Verification items for the finished model (mm, model axes). A direction names the side the tool comes from. Round coordinates to 2 decimals unless told otherwise and drop trailing zeros. Order: outer loops, then holes, each group sorted by start corner. A loop starts at its lowest first (then second) coordinate and runs counter-clockwise, first axis right, second up. Notation, with made-up numbers: (62, 58) -> (73, 58) arc R10 cw to (73, 72) -> close; hole circle Ø7 at (-38.5, -31.75). An arc over 180 degrees is marked (long way). Put each result on its own line as item: value.
```python
from build123d import *

# Parameters (mm, degrees)
SKETCH2_R           = 6.858
EXTRUDE1_DEPTH      = 13.273264
EXTRUDE1_DRAFT      = -1.783333333
CHAMFER1_SIZE       = 1.002631579
CHAMFER1_SIZE2      = 1.035353254
SKETCH5_R           = 5.1435
EXTRUDE2_DEPTH      = 13.273264
EXTRUDE2_TAPER      = 1.783333333
CHAMFER2_SIZE       = 0.705555556
CHAMFER2_SIZE_2     = 0.728581919
EXTRUDE3_DEPTH      = 3.792361
EXTRUDE3_DEPTH_BACK = 3.792361
SKETCH10_OUTSIDE_W  = 118.396
SKETCH10_OUTSIDE_H  = 121.158
SKETCH10_OUTSIDE_R  = 8.9296875
CUT_EXTRUDE1_DEPTH  = 25.922158813
CUT_EXTRUDE1_DRAFT  = -60
SKETCH11_OUTSIDE_W  = 118.396
SKETCH11_OUTSIDE_H  = 121.158
SKETCH11_OUTSIDE_R  = 8.9296875
CUT_EXTRUDE2_DEPTH  = 25.922158813
CUT_EXTRUDE2_DRAFT  = -60
SKETCH12_R          = 4.6228
CUT_EXTRUDE3_DEPTH  = 13.273265
SKETCH13_R          = 3.4163
CUT_EXTRUDE4_DEPTH  = 37.75596067


with BuildPart() as part:
    # Sketch2 → Extrude1 (with draft: the straight prism first)
    with BuildSketch(Plane(origin=(-3.792361111, 0, 0), x_dir=(0, 0, -1), z_dir=(1, 0, 0))):
        Circle(SKETCH2_R)
    extrude(amount=-EXTRUDE1_DEPTH)
    # Extrude1: the draft: its side faces are tilted about the plane it starts from
    extrude1_sides = [part.faces().sort_by_distance(p)[0] for p in [
        (-10.428993111, 0, 6.858),
    ]]
    draft(extrude1_sides, Plane(origin=(-3.792361111, 0, 0), x_dir=(0, 0, -1), z_dir=(1, 0, 0)), EXTRUDE1_DRAFT)

    # Chamfer1
    chamfer1_edges = [part.edges().sort_by_distance(p)[0] for p in [
        (-17.065625111, 0, 6.444735688),
    ]]
    chamfer1_side = [part.faces().sort_by_distance(p)[0] for p in [
        (-17.065625111, 0, 0),
    ]]
    chamfer(chamfer1_edges, length=CHAMFER1_SIZE, length2=CHAMFER1_SIZE2, reference=chamfer1_side[0])



with BuildPart() as body_2:
    # Sketch5 → Extrude2 (new body)
    with BuildSketch(Plane(origin=(3.792361111, 0, 0), x_dir=(0, 0, -1), z_dir=(1, 0, 0))):
        Circle(SKETCH5_R)
    extrude(amount=EXTRUDE2_DEPTH, taper=EXTRUDE2_TAPER)

    # Chamfer2
    # the kernel refuses this chamfer: 0.728581919, 0.705555556 mm, written as the material it takes off along each edge
    with BuildSketch(Plane(origin=(17.065625111, 0, 0), x_dir=(0, 0, -1), z_dir=(0, 1, 0))) as chamfer2_piece_1:
        Polygon((4.730235688 + CHAMFER2_SIZE * 0.0311200130608, CHAMFER2_SIZE * 0.999515654468), (4.730235688 - CHAMFER2_SIZE_2, 0), (4.730235688, 0), align=None)
    revolve(axis=Axis((17.065625111, 0, 0), (-1, 0, 0)), mode=Mode.SUBTRACT)


with BuildPart() as part_1:
    add(part.part)

    add(body_2.part)  # Revolve1 merges body 2
    # Sketch8 → Revolve1 (revolve)
    with BuildSketch(Plane.XY, mode=Mode.PRIVATE) as revolve1_sk:
        Polygon((0, 6.858), (-3.792361111, 6.858), (-10.476571637, 5.066971187), (-10.476571637, 0), (10.476571637, 0), (10.476571637, 3.352471187), (3.792361111, 5.1435), (0, 5.1435), align=None)
    revolve(revolve1_sk.sketch.rotate(Axis((-17.065625, 0, 0), (1, 0, 0)), 90), axis=Axis((-17.065625, 0, 0), (1, 0, 0)))

    # Sketch9 → Extrude3 (add, two sides: drawn at the far end of the back side and taken through both)
    with BuildSketch(Plane(origin=(0, 0, 0), x_dir=(0, 0, -1), z_dir=(1, 0, 0)).offset(-EXTRUDE3_DEPTH_BACK)):
        Polygon((0, 10.311114964), (-8.9296875, 5.155557482), (-8.9296875, -5.155557482), (0, -10.311114964), (8.9296875, -5.155557482), (8.9296875, 5.155557482), align=None)
    extrude(amount=EXTRUDE3_DEPTH + EXTRUDE3_DEPTH_BACK)


with BuildPart() as cut_extrude1_tool:
    # Sketch10 outside → Cut-Extrude1 (with draft: the straight prism first)
    with BuildSketch(Plane(origin=(3.792361111, 0, 0), x_dir=(0, 0, -1), z_dir=(1, 0, 0))):
        Rectangle(SKETCH10_OUTSIDE_W, SKETCH10_OUTSIDE_H)
        Circle(SKETCH10_OUTSIDE_R, mode=Mode.SUBTRACT)
    extrude(amount=-CUT_EXTRUDE1_DEPTH)
    # Cut-Extrude1: the draft: its side faces are tilted about the plane it starts from
    cut_extrude1_sides = [cut_extrude1_tool.faces().sort_by_distance(p)[0] for p in [
        (-9.168718295, -60.579, 0),
        (-9.168718295, 0, -59.198),
        (-9.168718295, 60.579, 0),
        (-9.168718295, 0, 59.198),
        (-9.168718295, 0, 8.9296875),
    ]]
    draft(cut_extrude1_sides, Plane(origin=(3.792361111, 0, 0), x_dir=(0, 0, -1), z_dir=(1, 0, 0)), CUT_EXTRUDE1_DRAFT)


with BuildPart() as part_2:
    add(part_1.part)

    # Cut-Extrude1: cut by cut_extrude1_tool
    add(cut_extrude1_tool.part, mode=Mode.SUBTRACT)


with BuildPart() as cut_extrude2_tool:
    # Sketch11 outside → Cut-Extrude2 (with draft: the straight prism first)
    with BuildSketch(Plane.ZY.offset(3.792361111)):
        Rectangle(SKETCH11_OUTSIDE_W, SKETCH11_OUTSIDE_H)
        Circle(SKETCH11_OUTSIDE_R, mode=Mode.SUBTRACT)
    extrude(amount=-CUT_EXTRUDE2_DEPTH)
    # Cut-Extrude2: the draft: its side faces are tilted about the plane it starts from
    cut_extrude2_sides = [cut_extrude2_tool.faces().sort_by_distance(p)[0] for p in [
        (9.168718295, -60.579, 0),
        (9.168718295, 0, 59.198),
        (9.168718295, 60.579, 0),
        (9.168718295, 0, -59.198),
        (9.168718295, 0, -8.9296875),
    ]]
    draft(cut_extrude2_sides, Plane.ZY.offset(3.792361111), CUT_EXTRUDE2_DRAFT)


with BuildPart() as part_3:
    add(part_2.part)

    # Cut-Extrude2: cut by cut_extrude2_tool
    add(cut_extrude2_tool.part, mode=Mode.SUBTRACT)

    # Sketch12 → Cut-Extrude3 (cut)
    with BuildSketch(Plane.ZY.offset(17.065625)):
        Circle(SKETCH12_R)
    extrude(amount=-CUT_EXTRUDE3_DEPTH, mode=Mode.SUBTRACT)

    # Sketch13 → Cut-Extrude4 (cut, through all)
    with BuildSketch(Plane(origin=(17.065625, 0, 0), x_dir=(0, 0, -1), z_dir=(1, 0, 0))):
        Circle(SKETCH13_R)
    extrude(amount=-CUT_EXTRUDE4_DEPTH, mode=Mode.SUBTRACT)

    # Cut-Extrude5 cone 1 section (through the dimple's axis) → Cut-Extrude5 (revolve, cut)
    with BuildSketch(Plane(origin=(-3.792361111, 0, 0), x_dir=(0, 0, 1), z_dir=(0, 1, 0))):
        Polygon((0, 0), (4.6228, 0), (0, 5.317923073), align=None)
    revolve(axis=Axis((-3.792361111, 0, 0), (1, 0, 0)), mode=Mode.SUBTRACT)


solid = part_3.part
```
Item 1: Release check for a two-part mould opening along Y. For faces 3 (the face through (-3.6, -9.26, -0.02)), 4 (the face through (-3.6, 4.61, 8.03)), 5 (the face through (-10.52, -2.81, -3.67)) record: pulls with the +Y half, pulls with the -Y half, needs draft (parallel to the pull), parting line crosses it, or undercut.
Geometry check:
face 3: pulls with the -Y half
face 4: pulls with the +Y half
face 5: undercut
Item 2: Depth check by flat-ended pin: pin 1 Ø8 at (y, z) = (5, -5) entering from -X; pin 2 Ø8 at (y, z) = (0, 0) entering from -X; pin 3 Ø1.5 at (x, z) = (5, -1.5) entering from -Y; pin 4 Ø3 at (x, z) = (-5, 6) entering from +Y. Enter the tip coordinate at first touch or a pass-through.
Geometry check:
pin 1: x = -17.07
pin 2: x = -3.08
pin 3: y = -5.05
pin 4: y = 7.35
Item 3: Material ranges on line 1 along Y through (x, z) = (2, 0); line 2 along Z through (x, y) = (4, 0); line 3 along X through (y, z) = (2.75, 7), recorded low to high.
Geometry check:
line 1: -10.31 to -3.42, 3.42 to 10.31
line 2: -5.14 to -3.42, 3.42 to 5.14
line 3: -3.79 to 3.79
Item 4: Tool access check on faces 1 (the face through (3.792, -4, -4)), 2 (the face through (0, 8, 4)). Record the directions out of +Z, -Z, +X, -X, +Y, -Y that give a thin tool (end or side, any length) a straight path to the whole face; none if there is none.
Geometry check:
face 1: +X
face 2: +Z, +X, -X, +Y
Item 5: Sectioned sample at A-A, the plane x = -1.5. Record the boundary of the cut face in (y, z), then the cut area to 3 significant figures.
Geometry check:
outline: (-10.31, 0) -> (-5.16, -8.93) -> (5.16, -8.93) -> (10.31, 0) -> (5.16, 8.93) -> (-5.16, 8.93) -> close; hole circle Ø6.83 at (0, 0)
area: 240 mm2
Item 6: Sectioned sample at B-B, the plane x = -9.5. Record the boundary of the cut face in (y, z).
Geometry check:
outline: circle Ø13.36 at (0, 0); hole circle Ø9.25 at (0, 0)
